Could you check a few things on this drawing? It's one solid part, dimensions in mm from its lowest x, y, z. A direction names the side the tool comes from. Give positions to 0.01 mm unless a question says otherwise; leave off trailing zeros. Write each loop counter-clockwise with the first axis right and the second up, starting at its lowest first coordinate (ties: lowest second). Pieces come first, ordered by that corner, then holes. Notation, with made-up numbers: M -29,-12.75 L -2,-12.75 A14 cw -2,-6.75 Z; hole C -24,7 d4. An arc over 180 degrees is marked long. Write each question's results on one line, items separated by ' | '.
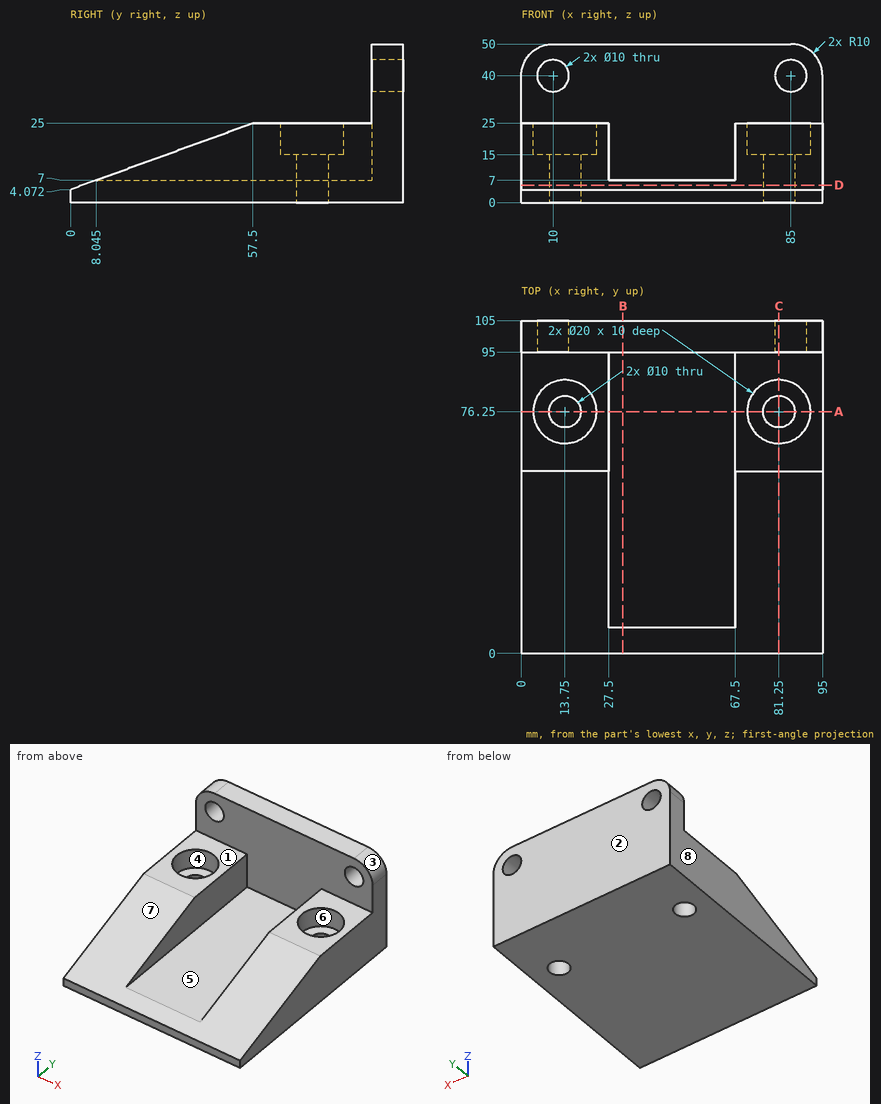
Item 1: For the marked faces 1, 2, 3, 4 and 5, which set-ups out of +Z, -Z, +X, -X, +Y, -Y let a thin tool reach every point of the face, with its end or its side?
Geometry says:
face 1: +Z, +X, -X, -Y | face 2: +Z, -Z, +X, -X, +Y | face 3: +Z, +X, +Y, -Y | face 4: +Z | face 5: +Z, -Y
Item 2: I want a section at B-B, the plane x = 32. Please give me the cut outline in (y, z) (1 decimal), and give its area (3 significant figures).
Geometry says:
outline: M 0,0 L 105,0 L 105,50 L 95,50 L 95,7 L 8,7 L 0,4.1 Z | area: 1,150 mm2
Item 3: I want a section at D-D, the plane z = 5.5. Give the number of separate pieces and of enclosed holes in the cut face.
Geometry says:
separate pieces: 1 | enclosed holes: 2
Item 4: I'm going to push flat-ended pins straight in: pin 1 (14 mm diameter, centred on x = 78, y = 74.5, fed in from +Z); pin 2 (3 mm diameter, centred on x = 25.5, y = 26, fed in from +Z); pin 3 (16 mm diameter, centred on x = 81.25, y = 76.25, fed in from +Z). Where does each tip first touch, or does it pass through?
Geometry says:
pin 1: stops at z = 25 | pin 2: stops at z = 14.08 | pin 3: stops at z = 15
Item 5: If I drill on line 1 (X direction, y = 76, z = 23); line 2 (X direction, y = 76, z = 9); line 3 (X direction, y = 93.5, z = 10.5), over which ranges is the centre line in solid material (lowest first)? Write a range as from..to.
Geometry says:
line 1: x = 0..3.75, 23.75..27.5, 67.5..71.25, 91.25..95 | line 2: x = 0..8.76, 18.74..27.5, 67.5..76.26, 86.24..95 | line 3: x = 0..27.5, 67.5..95
Item 6: Thinking about a two-plate mould opening in Y: for the marked faces 6, 7 and 8, which applies, +Y half, -Y half, draft (parallel to the pull), parting line (faces both ways), or undercut?
Geometry says:
face 6: undercut | face 7: -Y half | face 8: draft
Item 7: I want a section at A-A, the plane y = 76.25. Please give me the cut outline in (x, z).
Geometry says:
outline: M 0,0 L 8.75,0 L 8.75,15 L 3.75,15 L 3.75,25 L 0,25 Z; M 18.75,0 L 76.25,0 L 76.25,15 L 71.25,15 L 71.25,25 L 67.5,25 L 67.5,7 L 27.5,7 L 27.5,25 L 23.75,25 L 23.75,15 L 18.75,15 Z; M 86.25,0 L 95,0 L 95,25 L 91.25,25 L 91.25,15 L 86.25,15 Z
Item 8: I want a section at C-C, the plane x = 81.25. Please give me the cut outline in (y, z), and give its area (3 significant figures).
Geometry says:
outline: M 0,0 L 71.25,0 L 71.25,15 L 66.25,15 L 66.25,25 L 57.5,25 L 0,4.07 Z; M 81.25,0 L 105,0 L 105,36.69 L 95,36.69 L 95,25 L 86.25,25 L 86.25,15 L 81.25,15 Z; M 95,43.31 L 105,43.31 L 105,50 L 95,50 Z | area: 1,860 mm2
